from build123d import *

# Parameters (mm, degrees)
F0_R      = 12
F1_DEPTH  = 8
F2_R      = 10
F3_DEPTH  = 10
F4_R      = 9
F5_DEPTH  = 6
F6_W      = 1
F6_H      = 2
F9_SIZE   = 1
F10_SIZE  = 0.99999
F11_R     = 6
F12_DEPTH = 42.1


# Not quite as in the source:
# - a fillet or chamfer is up to 0.001 mm smaller than in the source, because OpenCascade refuses the exact size


with BuildPart() as f1:
    # F0 (on Top) → F1 (new body)
    with BuildSketch(Plane.XY):
        Circle(F0_R)
    extrude(amount=F1_DEPTH)

    # F2 (on face) → F3 (join)
    with BuildSketch(Plane.XY.offset(8)):
        Circle(F2_R)
    extrude(amount=F3_DEPTH)

    # F4 (on face) → F5 (join)
    with BuildSketch(Plane.XY.offset(18)):
        Circle(F4_R)
    extrude(amount=F5_DEPTH)

    # F6 (on Right) → F8 (revolve, cut)
    with BuildSketch(Plane.YZ):
        with Locations((9.5, 9)):
            Rectangle(F6_W, F6_H)
    revolve(axis=Axis((0, 0, 13.7254064903), (0, 0, 1)), mode=Mode.SUBTRACT)

    # F9
    f9_edges = [f1.edges().sort_by_distance(p)[0] for p in [
        (-12, 0, 0),
    ]]
    chamfer(f9_edges, length=F9_SIZE)

    # F10 (size 1 in the source; OpenCascade refuses exactly that, so slightly less here)
    f10_edges = [f1.edges().sort_by_distance(p)[0] for p in [
        (-10, 0, 18),
    ]]
    chamfer(f10_edges, length=F10_SIZE)

    # F11 (on face) → F12 (cut)
    with BuildSketch(Plane.XY.offset(24)):
        Circle(F11_R)
    extrude(amount=-F12_DEPTH, mode=Mode.SUBTRACT)


solid = f1.part
Work out the finished part from the listing and answer in its coordinate system (mm). A direction names the side the tool comes from. Round coordinates to 2 decimals unless told otherwise and drop trailing zeros. Order: outer loops, then holes, each group sorted by start corner. A loop starts at its lowest first (then second) coordinate and runs counter-clockwise, first axis right, second up. Notation, with made-up numbers: M 71.25,-16.5 L 84.25,-16.5 A20 cw 84.25,4.5 Z; hole C 51,17.25 d2. An arc over 180 degrees is marked long. One line per item, written item: value.
Q1. Flat-ended cylindrical pins translate along their axes: pin 1 (2 mm diameter, centred on y = 9, z = 14.5, fed in from +X); pin 2 (6 mm diameter, centred on x = -0.5, y = -1.5, fed in from -Z); pin 3 (1 mm diameter, centred on y = 4, z = 10, fed in from -X); pin 4 (6 mm diameter, centred on y = 5, z = 12.5, fed in from -X). Find the tip coordinate at first contact, or state that the pin passes through.
Derived:
pin 1: x = 6
pin 2: through
pin 3: x = -9.37
pin 4: x = -9.8
Q2. Find section B-B on z = 15.25. Write down the section's boundary in (x, y).
Derived:
outline: C 0,0 d20; hole C 0,0 d12
Q3. For faces 4 (the face through (-8.923, -1.172, 9.014)), 5 (the face through (2, -6, 24)), 6 (the face through (9.54, 3, 13.45)), determine the directions among +Z, -Z, +X, -X, +Y, -Y from which every point of the face is accessible in a straight line to the end or side of a thin tool.
Derived:
face 4: none
face 5: +Z, +X, -X, +Y, -Y
face 6: +Z
Q4. Find section C-C on z = 2.25. Write down the section's boundary in (x, y), then the cut area to 3 significant figures.
Derived:
outline: C 0,0 d24; hole C 0,0 d12
area: 339 mm²
Q5. Straight lines are drawn through the part: line 1 (Y direction, x = 0, z = 18); line 2 (Z direction, x = 9, y = 4.75); line 3 (Y direction, x = -3, z = 2.5). For each, find the intervals that lie inside material, in ascending order.
Derived:
line 1: -9 to -6, 6 to 9
line 2: 0 to 8
line 3: -11.62 to -5.2, 5.2 to 11.62
Q6. Determine the mould class of faces 1 (the face through (5, -5, 0)), 2 (the face through (-2, 9, 10)), 3 (the face through (-11.99, 0.53, 4.45)) for opening direction Z: released by +Z, released by -Z, zero draft, split by the parting line, or undercut.
Derived:
face 1: released by -Z
face 2: undercut
face 3: zero draft
